```python
from build123d import *

# Parameters (mm, degrees)
SKETCH1_R            = 1.8
BOSS_EXTRUDE1_DEPTH  = 20
CUT_EXTRUDE1_DEPTH   = 6.5
CUT_EXTRUDE2_DEPTH   = 5
MIRROR2_COPY_1_DEPTH = 6.5


with BuildPart() as part:
    # Sketch1 → Boss-Extrude1 (new body)
    with BuildSketch(Plane(origin=(0, 0, 0), x_dir=(0, 0, -1), z_dir=(1, 0, 0))):
        Circle(SKETCH1_R)
    extrude(amount=BOSS_EXTRUDE1_DEPTH)

    # Sketch2 → Cut-Extrude1 (cut)
    with BuildSketch(Plane(origin=(20, 0, 0), x_dir=(0, 0, -1), z_dir=(1, 0, 0))):
        with BuildLine():
            Line((-1, 0), (-1.8, 0))
            ThreePointArc((-1.8, 0), (0, 1.8), (1.8, 0))
            Line((1.8, 0), (1, 0))
            ThreePointArc((1, 0), (0, 1), (-1, 0))
        make_face()
    cut_extrude1 = extrude(amount=-CUT_EXTRUDE1_DEPTH, mode=Mode.SUBTRACT)

    # Sketch3 → Cut-Extrude2 (cut)
    with BuildSketch(Plane(origin=(12.5, 0, 0), x_dir=(0, 0, -1), z_dir=(1, 0, 0))):
        with BuildLine():
            Line((-1, 0), (-1.8, 0))
            ThreePointArc((-1.8, 0), (0, 1.8), (1.8, 0))
            Line((1.8, 0), (1, 0))
            ThreePointArc((1, 0), (0, 1), (-1, 0))
        make_face()
    cut_extrude2 = extrude(amount=-CUT_EXTRUDE2_DEPTH, mode=Mode.SUBTRACT)

    # Mirror1: Cut-Extrude1 across plane
    add(cut_extrude1.mirror(Plane(origin=(10, 0, 0), x_dir=(0, 0, 1), z_dir=(1, 0, 0))), mode=Mode.SUBTRACT)

    # Mirror2: Cut-Extrude2, Cut-Extrude1 across plane
    add(cut_extrude2.mirror(Plane.ZX), mode=Mode.SUBTRACT)
    add(cut_extrude1.mirror(Plane.ZX), mode=Mode.SUBTRACT)

    # Mirror2 copy 1 sketch → Mirror2 copy 1 (cut)
    with BuildSketch(Plane(origin=(0, 0, 0), x_dir=(0, 0, -1), z_dir=(-1, 0, 0))):
        with BuildLine():
            Line((-1, 0), (-1.8, 0))
            ThreePointArc((-1.8, 0), (0, 1.8), (1.8, 0))
            Line((1.8, 0), (1, 0))
            ThreePointArc((1, 0), (0, 1), (-1, 0))
        make_face()
    extrude(amount=-MIRROR2_COPY_1_DEPTH, mode=Mode.SUBTRACT)


solid = part.part
```
Build history of the part. All positions in model axes, mm. A direction names the side the tool comes from. Round coordinates to 2 decimals unless told otherwise and drop trailing zeros. Loops run counter-clockwise (first coordinate to the right, second up) from the corner with the lowest first, then second, coordinate; pieces in that order, holes last.
Item 1: Which spindle directions (+Z, -Z, +X, -X, +Y, -Y) get a long thin tool onto all of the face, cutting with end or side? Do faces 1 (the face through (13.5, -1, 1)), 2 (the face through (3, 1, 0)), 3 (the face through (12.5, -1, 1)). Say none if no direction does.
Item 2: Saw through at C-C (z = 1.2). List the corners of the cut face in (x, y), then the cut area to 3 significant figures.
Item 3: Pin check, flat tips, straight feed: P1, Ø1.5, axis at x = 11.5, y = -1.5, coming from the +Z side; P2, Ø1, axis at x = 3, z = 0.5, coming from the -Y side. Stop position of each tip, or through.
Item 4: Two-plate mould, pull along X, no slides. Class faces 4 (the face through (0, 0, 0)), 5 (the face through (7.5, 1, 1)), 6 (the face through (17, -1, 0)): released by +X, released by -X, zero draft, split by the parting line, or undercut.
Item 5: Saw through at B-B (y = -1.45). List the corners of the cut face in (x, z).
Item 6: Drill centre lines: line 1 along X through (y, z) = (1.5, 0.7); line 2 along Y through (x, z) = (9.5, 0.05); line 3 along Y through (x, z) = (9.75, -0.5). Where is each one in solid material? Low to high.
Item 7: Saw through at A-A (z = 0). List the corners of the cut face in (x, y), then the cut area to 3 significant figures.
Worked answers:
1. face 1: +X
1. face 2: -X
1. face 3: none
2. outline: (6.5, -1.34) - (7.5, -1.34) - (7.5, 1.34) - (6.5, 1.34) - close; (12.5, -1.34) - (13.5, -1.34) - (13.5, 1.34) - (12.5, 1.34) - close
2. area: 5.37 mm2
3. P1: stops at z = 0.66
3. P2: stops at y = -1
4. face 4: released by -X
4. face 5: undercut
4. face 6: zero draft
5. outline: (6.5, -1.07) - (7.5, -1.07) - (7.5, 1.07) - (6.5, 1.07) - close; (12.5, -1.07) - (13.5, -1.07) - (13.5, 1.07) - (12.5, 1.07) - close
6. line 1: x = 6.5 to 7.5, 12.5 to 13.5
6. line 2: y = -1 to 1
6. line 3: y = -0.87 to 0.87
7. outline: (0, -1) - (6.5, -1) - (6.5, -1.8) - (7.5, -1.8) - (7.5, -1) - (12.5, -1) - (12.5, -1.8) - (13.5, -1.8) - (13.5, -1) - (20, -1) - (20, 1) - (13.5, 1) - (13.5, 1.8) - (12.5, 1.8) - (12.5, 1) - (7.5, 1) - (7.5, 1.8) - (6.5, 1.8) - (6.5, 1) - (0, 1) - close
7. area: 43.2 mm2
